```python
from build123d import *

# Parameters (mm, degrees)
SKETCH1_W                = 82.55
SKETCH1_H                = 43.434
BOSS_EXTRUDE1_DEPTH      = 5.334
CUT_EXTRUDE1_START       = -88.085249325
CUT_EXTRUDE1_OUTLINE_W   = 5.334
CUT_EXTRUDE1_OUTLINE_H   = 5.334
CUT_EXTRUDE1_DEPTH       = 16.51
CUT_EXTRUDE1_START_2     = -55.065249325
CUT_EXTRUDE1_2_OUTLINE_W = 5.334
CUT_EXTRUDE1_2_OUTLINE_H = 5.334
CUT_EXTRUDE1_2_DEPTH     = 16.51
CUT_EXTRUDE1_START_3     = -22.045249325
CUT_EXTRUDE1_3_OUTLINE_W = 5.334
CUT_EXTRUDE1_3_OUTLINE_H = 5.334
CUT_EXTRUDE1_3_DEPTH     = 16.51
SKETCH3_W                = 5.334
SKETCH3_H                = 9.638319844
SKETCH3_H_2              = 9.638319843
CUT_EXTRUDE2_DEPTH       = 93.990910348
SKETCH4_R                = 12.7
CUT_EXTRUDE3_DEPTH       = 93.990910348


# Read off the part's stored shape, not the designer's step: Cut-Extrude1
with BuildPart() as part:
    # Sketch1 → Boss-Extrude1 (new body)
    with BuildSketch(Plane.XY):
        with Locations((-46.810249325, -7.606142782)):
            Rectangle(SKETCH1_W, SKETCH1_H)
    extrude(amount=BOSS_EXTRUDE1_DEPTH)

    # Cut-Extrude1 outline → Cut-Extrude1 (cut)
    with BuildSketch(Plane.YZ.offset(CUT_EXTRUDE1_START)):
        with Locations((11.443857218, 2.667)):
            Rectangle(CUT_EXTRUDE1_OUTLINE_W, CUT_EXTRUDE1_OUTLINE_H)
    extrude(amount=CUT_EXTRUDE1_DEPTH, mode=Mode.SUBTRACT)

    # Cut-Extrude1 2 outline → Cut-Extrude1 2 (cut)
    with BuildSketch(Plane.YZ.offset(CUT_EXTRUDE1_START_2)):
        with Locations((11.443857218, 2.667)):
            Rectangle(CUT_EXTRUDE1_2_OUTLINE_W, CUT_EXTRUDE1_2_OUTLINE_H)
    extrude(amount=CUT_EXTRUDE1_2_DEPTH, mode=Mode.SUBTRACT)

    # Cut-Extrude1 3 outline → Cut-Extrude1 3 (cut)
    with BuildSketch(Plane.YZ.offset(CUT_EXTRUDE1_START_3)):
        with Locations((11.443857218, 2.667)):
            Rectangle(CUT_EXTRUDE1_3_OUTLINE_W, CUT_EXTRUDE1_3_OUTLINE_H)
    extrude(amount=CUT_EXTRUDE1_3_DEPTH, mode=Mode.SUBTRACT)

    # Sketch3 → Cut-Extrude2 (cut, through all)
    with BuildSketch(Plane.XY.offset(5.334)):
        with Locations((-85.418249325, -24.50398286)):
            Rectangle(SKETCH3_W, SKETCH3_H)
        with Locations((-85.418249325, -5.227343173)):
            Rectangle(SKETCH3_W, SKETCH3_H_2)
        with Locations((-8.202249325, -24.50398286)):
            Rectangle(SKETCH3_W, SKETCH3_H)
        with Locations((-8.202249325, -5.227343173)):
            Rectangle(SKETCH3_W, SKETCH3_H_2)
    extrude(amount=-CUT_EXTRUDE2_DEPTH, mode=Mode.SUBTRACT)

    # Sketch4 → Cut-Extrude3 (cut, through all)
    with BuildSketch(Plane.XY.offset(5.334)):
        with Locations((-46.810249325, -3.923396782)):
            Circle(SKETCH4_R)
    extrude(amount=-CUT_EXTRUDE3_DEPTH, mode=Mode.SUBTRACT)


solid = part.part
```
Design review of the part built by this model. Coordinates are the model's own, in mm. A direction names the side the tool comes from. Round coordinates to 2 decimals unless told otherwise and drop trailing zeros. Order: outer loops, then holes, each group sorted by start corner. A loop starts at its lowest first (then second) coordinate and runs counter-clockwise, first axis right, second up. Notation, with made-up numbers: M 5.5,63.5 L 32.5,63.5 A24 cw 32.5,93.5 Z; hole C 2.25,89.25 d7. An arc over 180 degrees is marked long. Put each result on its own line as item: value.
Q1. Insertion check: pin 1 Ø1.6 at (y, z) = (11, 3) entering from +X; pin 2 Ø1.6 at (y, z) = (12, 1.5) entering from -X; pin 3 Ø2.5 at (y, z) = (-3.5, 2.5) entering from -X; pin 4 Ø10 at (x, y) = (-40, -0.5) entering from -Z. Each pin has a flat end and moves straight along its axis. Give the tip position at first contact, or say it passes through.
Reported:
pin 1: x = -22.05
pin 2: x = -71.58
pin 3: x = -82.75
pin 4: through
Q2. Consider section A-A (x = -40). State the section outline as (y, z) points.
Reported:
outline: M -29.32,0 L -14.64,0 L -14.64,5.33 L -29.32,5.33 Z; M 6.8,0 L 8.78,0 L 8.78,5.33 L 6.8,5.33 Z
Q3. Consider section B-B (y = 4.5). State the section outline as (x, z) points.
Reported:
outline: M -88.09,0 L -56.31,0 L -56.31,5.33 L -88.09,5.33 Z; M -37.31,0 L -5.54,0 L -5.54,5.33 L -37.31,5.33 Z
Q4. Consider section C-C (z = 4.5). State the section outline as (x, y) points.
Reported:
outline: M -88.09,-19.68 L -82.75,-19.68 L -82.75,-29.32 L -10.87,-29.32 L -10.87,-19.68 L -5.54,-19.68 L -5.54,-10.05 L -10.87,-10.05 L -10.87,-0.41 L -5.54,-0.41 L -5.54,8.78 L -22.05,8.78 L -22.05,14.11 L -38.56,14.11 L -38.56,8.78 L -55.07,8.78 L -55.07,14.11 L -71.58,14.11 L -71.58,8.78 L -88.09,8.78 L -88.09,-0.41 L -82.75,-0.41 L -82.75,-10.05 L -88.09,-10.05 Z; hole C -46.81,-3.92 d25.4
Q5. To check wall thickness, follow line 1 (X direction, y = 9.5, z = 5.1); line 2 (X direction, y = -24, z = 1.9); line 3 (X direction, y = 7, z = 1.95). State the ranges of each line that lie inside material, in increasing order.
Reported:
line 1: -71.58 to -55.07, -38.56 to -22.05
line 2: -82.75 to -10.87
line 3: -88.09 to -53.29, -40.33 to -5.54
Q6. Machinability: for faces 5 (the face through (-82.751, -5, 3)), 6 (the face through (-14, 8.777, 3)), 7 (the face through (-8, -0.408, 3)), which of the approach directions +Z, -Z, +X, -X, +Y, -Y give a long, thin tool a straight path to every point of the face, cutting with its end or side? Answer none if there is none.
Reported:
face 5: +Z, -Z, -X
face 6: +Z, -Z, +X, +Y
face 7: +Z, -Z, +X
Q7. Draft analysis for pull direction X (two halves, no side actions). For faces 1 (the face through (-10.869, -25, 3)), 2 (the face through (-55.065, 11, 3)), 3 (the face through (-8, -19.685, 3)), 4 (the face through (-82.751, -25, 3)), state which applies: released by +X, released by -X, zero draft, split by the parting line, or undercut.
Reported:
face 1: released by +X
face 2: undercut
face 3: zero draft
face 4: released by -X
Q8. Consider section D-D (x = -13.5). State the section outline as (y, z) points, and give its area (3 significant figures).
Reported:
outline: M -29.32,0 L 8.78,0 L 8.78,5.33 L -29.32,5.33 Z
area: 203 mm²
